```python
from build123d import *

# Parameters (mm, degrees)
F1_DEPTH = 3.9
F2_DEPTH = 11.9
F3_DEPTH = 42.5


with BuildPart() as f1:
    # F0 (on Top) → F1 (new body)
    with BuildSketch(Plane.XY):
        with BuildLine():
            Line((15.2110805884, -1.0073357602), (1.2110805884, -1.0073357602))
            Line((1.2110805884, -1.0073357602), (1.2110805884, -8.5073357602))
            add(Edge.make_bspline(
                [(15.2110805884, -1.0073357602), (10.1056651112, -3.7045784545), (6.4222975956, -8.6121569817), (1.2110805884, -8.5073357602)],
                knots=[0.5948688465, 0.5948688465, 0.5948688465, 0.5948688465, 0.7145243028, 0.7145243028, 0.7145243028, 0.7145243028], degree=3))
        make_face()
        with BuildLine():
            Line((29.2110805884, -1.0073357602), (15.2110805884, -1.0073357602))
            add(Edge.make_bspline(
                [(15.2110805884, -1.0073357602), (10.1056651112, -3.7045784545), (6.4222975956, -8.6121569817), (1.2110805884, -8.5073357602)],
                knots=[0.5948688465, 0.5948688465, 0.5948688465, 0.5948688465, 0.7145243028, 0.7145243028, 0.7145243028, 0.7145243028], degree=3))
            Line((1.2110805884, -8.5073357602), (1.2110805884, -16.0073357602))
            add(Edge.make_bspline(
                [(1.2110805884, -16.0073357602), (1.5073310932, -15.9933259222), (1.7934505794, -15.9937789675), (2.0704529167, -16.0073357602)],
                knots=[0.1348057981, 0.1348057981, 0.1348057981, 0.1348057981, 0.1410104438, 0.1410104438, 0.1410104438, 0.1410104438], degree=3))
            Line((2.0704529167, -16.0073357602), (29.2110805884, -16.0073357602))
            Line((29.2110805884, -16.0073357602), (29.2110805884, -1.0073357602))
        make_face()
    extrude(amount=F1_DEPTH)

    # F0 (on Top) → F2 (join)
    with BuildSketch(Plane.XY):
        with BuildLine():
            Line((1.2110805884, -16.0073357602), (1.2110805884, -8.5073357602))
            add(Edge.make_bspline(
                [(1.2110805884, -8.5073357602), (-3.5186716625, -8.4121989798), (-9.506998743, -4.1880690008), (-11.1998226494, -4.3673282489)],
                knots=[0.7145243028, 0.7145243028, 0.7145243028, 0.7145243028, 0.823124782, 0.823124782, 0.823124782, 0.823124782], degree=3))
            Line((-11.1998226499, -4.367328249), (-11.1998226499, -20.0583143803))
            add(Edge.make_bspline(
                [(-11.1998226499, -20.0583143803), (-7.1868911838, -18.3499221531), (-2.2831850449, -16.1725813711), (1.2110805884, -16.0073357602)],
                knots=[0.0616221929, 0.0616221929, 0.0616221929, 0.0616221929, 0.1348057981, 0.1348057981, 0.1348057981, 0.1348057981], degree=3))
        make_face()
    extrude(amount=F2_DEPTH)

    # F0 (on Top) → F3 (join)
    with BuildSketch(Plane.XY):
        with BuildLine():
            Line((29.2110805884, -1.0073357602), (15.2110805884, -1.0073357602))
            add(Edge.make_bspline(
                [(15.2110805884, -1.0073357602), (10.1056651112, -3.7045784545), (6.4222975956, -8.6121569817), (1.2110805884, -8.5073357602)],
                knots=[0.5948688465, 0.5948688465, 0.5948688465, 0.5948688465, 0.7145243028, 0.7145243028, 0.7145243028, 0.7145243028], degree=3))
            Line((1.2110805884, -8.5073357602), (1.2110805884, -16.0073357602))
            add(Edge.make_bspline(
                [(1.2110805884, -16.0073357602), (1.5073310932, -15.9933259222), (1.7934505794, -15.9937789675), (2.0704529167, -16.0073357602)],
                knots=[0.1348057981, 0.1348057981, 0.1348057981, 0.1348057981, 0.1410104438, 0.1410104438, 0.1410104438, 0.1410104438], degree=3))
            Line((2.0704529167, -16.0073357602), (29.2110805884, -16.0073357602))
            Line((29.2110805884, -16.0073357602), (29.2110805884, -1.0073357602))
        make_face()
        with BuildLine():
            add(Edge.make_bspline(
                [(29.2110805884, -16.0073357602), (32.6593398461, -11.4234913165), (32.4818190242, -4.2330775311), (29.2110805884, -1.0073357602)],
                knots=[0.3662436292, 0.3662436292, 0.3662436292, 0.3662436292, 0.4825277311, 0.4825277311, 0.4825277311, 0.4825277311], degree=3))
            Line((29.2110805884, -1.0073357602), (29.2110805884, -16.0073357602))
        make_face()
        with BuildLine():
            add(Edge.make_bspline(
                [(2.0704529167, -16.0073357602), (6.535385921, -16.225854391), (11.2561235238, -24.3852753557), (25.4977786279, -20.9435071114), (29.2110805884, -16.0073357602)],
                knots=[0.1410104438, 0.1410104438, 0.1410104438, 0.1410104438, 0.2410216109, 0.3662436292, 0.3662436292, 0.3662436292, 0.3662436292], degree=3))
            Line((29.2110805884, -16.0073357602), (2.0704529167, -16.0073357602))
        make_face()
    extrude(amount=F3_DEPTH)


solid = f1.part
```
The model under review builds one solid part; all positions refer to its coordinate system, in mm. A direction names the side the tool comes from. Give positions to 0.01 mm unless a question says otherwise; leave off trailing zeros. Use CSV: the item, a comma, the result in double quotes.
1. To check wall thickness, follow probe 1 along Y at (x, z) = (16, 35); probe 2 along Z at (x, y) = (6.5, -4.5); probe 3 along Z at (x, y) = (-7, -12.25). State the ranges of each line that lie inside material, in increasing order. Write a range as from..to.
Result:
probe 1,"y = -21.77..-1.01"
probe 2,"z = 0..3.9"
probe 3,"z = 0..11.9"
2. Machinability: for faces 1 (the face through (10, -10, 0)), 2 (the face through (1.211, -5, 2)), 3 (the face through (-11.2, -12, 6)), 4 (the face through (7, -4, 3.9)), 5 (the face through (1.211, -12, 27)), which of the approach directions +Z, -Z, +X, -X, +Y, -Y give a long, thin tool a straight path to every point of the face, cutting with its end or side? Answer none if there is none.
Result:
face 1,"-Z, +X, -X, +Y, -Y"
face 2,"+Z, -Z, +Y"
face 3,"+Z, -Z, -X, +Y, -Y"
face 4,"+Z, +Y"
face 5,"+Z, -X, +Y, -Y"
3. For P1, Ø6, axis at y = -11, z = 17.5, coming from the -X side; P2, Ø10, axis at x = -6.5, y = -13.5, coming from the +Z side; P3, Ø10, axis at x = 26, z = 8, coming from the -Y side, all flat-tipped, find the tip position at first contact; note any pin that passes through.
Result:
P1,"stops at x = 1.21"
P2,"stops at z = 11.9"
P3,"stops at y = -21.18"
